from build123d import *

# Parameters (mm, degrees)
EXTRUDE_1_DEPTH              = 2.5
HOLE_WIZARD_M3_1_D           = 2.5
HOLE_WIZARD_M3_1_CSINK_D     = 3.05
HOLE_WIZARD_M3_1_CSINK_ANGLE = 90
SKETCH_8_W                   = 27.92487284
SKETCH_8_H                   = 6.74765502
SKETCH_8_W_2                 = 35.307317085
SKETCH_8_H_2                 = 2.5392143
SKETCH_8_W_3                 = 43.206671158
EXTRUDE_2_DEPTH              = 6
SKETCH_9_W                   = 15
SKETCH_9_H                   = 12
EXTRUDE_3_DEPTH              = 10.5
SKETCH_10_W                  = 2.54775384
SKETCH_10_H                  = 5.1401971
CUT_EXTRUDE_1_DEPTH          = 10.5
SKETCH_12_W                  = 14
SKETCH_12_H                  = 10
EXTRUDE_4_DEPTH              = 10
SKETCH_13_W                  = 10
SKETCH_13_H                  = 10
SKETCH_13_R                  = 2.75
EXTRUDE_5_DEPTH              = 3.5
SKETCH_14_R                  = 2.75
CUT_EXTRUDE_3_DEPTH          = 8


with BuildPart() as part:
    # 草图1 → 凸台-拉伸1 (new body)
    with BuildSketch(Plane.XY):
        Polygon((-35.4452235, 28.536703393), (-35.4452235, -24.463296607), (30.5947765, -24.463296607), (30.5947765, -20.997866899), (34.409346792, -17.183296607), (34.409346792, 10.756703393), (30.5947765, 14.571273684), (30.5947765, 28.536703393), align=None)
    extrude(amount=EXTRUDE_1_DEPTH)

    # M3 螺纹孔1 (through all)
    with Locations(Plane.XY.offset(2.5)):
        with Locations((-20.2052235, 25.996703393), (30.5947765, 10.756703393), (30.5947765, -17.183296607), (-20.2052235, -22.263296607)):
            CounterSinkHole(HOLE_WIZARD_M3_1_D / 2, HOLE_WIZARD_M3_1_CSINK_D / 2, counter_sink_angle=HOLE_WIZARD_M3_1_CSINK_ANGLE)

    # 草图8 → 凸台-拉伸2 (add)
    with BuildSketch(Plane.XY.offset(2.5)):
        with Locations((7.351969456, -11.104054762)):
            Rectangle(SKETCH_8_W, SKETCH_8_H)
        with Locations((7.55461376, -21.179250047)):
            Rectangle(SKETCH_8_W_2, SKETCH_8_H_2)
        with Locations((5.71151473, 24.713414732)):
            Rectangle(SKETCH_8_W_3, SKETCH_8_H_2)
    extrude(amount=EXTRUDE_2_DEPTH)

    # 草图9 → 凸台-拉伸3 (add)
    with BuildSketch(Plane.XY.offset(2.5)):
        with Locations((-33.9452235, 12.536703393)):
            Rectangle(SKETCH_9_W, SKETCH_9_H)
    extrude(amount=EXTRUDE_3_DEPTH)

    # 草图10 → 切除-拉伸1 (cut)
    with BuildSketch(Plane.ZY.offset(41.4452235)):
        Polygon((3.5, 17.344772898), (3.5, 7.728633887), (9.323306646, 7.728633887), (12, 9.706966862), (12, 15.452627596), (9.323306646, 17.344772898), align=None)
        with Locations((7.507872917, 12.536703393)):
            Rectangle(SKETCH_10_W, SKETCH_10_H, mode=Mode.SUBTRACT)
    extrude(amount=-CUT_EXTRUDE_1_DEPTH, mode=Mode.SUBTRACT)

    # 草图12 → 凸台-拉伸4 (add)
    with BuildSketch(Plane.XY.offset(2.5)):
        with Locations((-28.4452235, -13.463296607)):
            Rectangle(SKETCH_12_W, SKETCH_12_H)
    extrude(amount=EXTRUDE_4_DEPTH)

    # 草图13 → 凸台-拉伸5 (add)
    with BuildSketch(Plane.ZY.offset(35.4452235)):
        with Locations((7.5, -13.463296607)):
            Rectangle(SKETCH_13_W, SKETCH_13_H)
        with Locations((7.5, -13.463296607)):
            Circle(SKETCH_13_R, mode=Mode.SUBTRACT)
    extrude(amount=EXTRUDE_5_DEPTH)

    # 草图14 → 切除-拉伸3 (cut)
    with BuildSketch(Plane.ZY.offset(35.4452235)):
        with Locations((7.5, -13.463296607)):
            Circle(SKETCH_14_R)
    extrude(amount=-CUT_EXTRUDE_3_DEPTH, mode=Mode.SUBTRACT)


solid = part.part
Read the model definition and answer for the solid it produces. Units are mm, in the model's axes. A direction names the side the tool comes from. Round coordinates to 2 decimals unless told otherwise and drop trailing zeros. Write each loop counter-clockwise with the first axis right and the second up, starting at its lowest first coordinate (ties: lowest second). Pieces come first, ordered by that corner, then holes.
1. The part is cut by section C-C, the plane z = 11.25. Determine the outline of the cut face in (x, y), then the cut area to 3 significant figures.
2. The part is cut by section A-A, the plane z = 7.5. State how many separate pieces and enclosed holes the cut face has, then the cut area to 3 significant figures.
3. Which of the six approach directions +Z, -Z, +X, -X, +Y, -Y give full straight-line access (tool end or side, diameter ignored) to faces 5 (the face through (-38.945, -11, 10)), 6 (the face through (-33.11, -14.52, 10.04)), 7 (the face through (-10.099, -21, 5)), 8 (the face through (-34, 6.537, 8))?
4. Determine the mould class of faces 1 (the face through (-30, -8.463, 7)), 2 (the face through (-38, 13, 2.5)), 3 (the face through (-36, 7.729, 6)), 4 (the face through (-36, 13, 3.5)) for opening direction Z: pulls with the +Z half, pulls with the -Z half, needs draft (parallel to the pull), parting line crosses it, or undercut.
5. Straight lines are drawn through the part: L1, parallel to Y at x = -31.5, z = 4.5; L2, parallel to Y at x = -32, z = 7.5; L3, parallel to Y at x = 3, z = 4. For each, find the intervals that lie inside material, in ascending order.
6. The part is cut by section B-B, the plane x = -2.5. Determine the outline of the cut face in (y, z).
7. Given pin 1 Ø6.5 at (x, z) = (13.5, 4) entering from -Y; pin 2 Ø1.3 at (y, z) = (-20.5, 6) entering from +X; pin 3 Ø3 at (x, z) = (9, 5.5) entering from +Y; pin 4 Ø3 at (y, z) = (22.5, 1) entering from +X, each flat-ended and moving along its own axis, determine where each tip first touches the part or whether it passes through.
8. The part is cut by section D-D, the plane y = -5. Determine the outline of the cut face in (x, z), then the cut area to 3 significant figures.
Values:
1. outline: (-41.45, 6.54) - (-26.45, 6.54) - (-26.45, 18.54) - (-41.45, 18.54) - (-41.45, 15.98) - (-30.95, 15.98) - (-30.95, 9.15) - (-41.45, 9.15) - close; (-38.95, -18.46) - (-21.45, -18.46) - (-21.45, -8.46) - (-38.95, -8.46) - close
1. area: 283 mm2
2. separate pieces: 5
2. enclosed holes: 0
2. area: 633 mm2
3. face 5: +Z, -Z, -X, -Y
3. face 6: -X
3. face 7: +Z, -X, -Y
3. face 8: +Z, +X, -X
4. face 1: needs draft
4. face 2: pulls with the -Z half
4. face 3: undercut
4. face 4: undercut
5. L1: y = -18.46 to -8.46, 6.54 to 7.73, 17.34 to 18.54
5. L2: y = -18.46 to -16.21, -10.71 to -8.46, 6.54 to 7.73, 9.97 to 15.11, 17.34 to 18.54
5. L3: y = -22.45 to -19.91, -14.48 to -7.73, 23.44 to 25.98
6. outline: (-24.46, 0) - (28.54, 0) - (28.54, 2.5) - (25.98, 2.5) - (25.98, 8.5) - (23.44, 8.5) - (23.44, 2.5) - (-7.73, 2.5) - (-7.73, 8.5) - (-14.48, 8.5) - (-14.48, 2.5) - (-19.91, 2.5) - (-19.91, 8.5) - (-22.45, 8.5) - (-22.45, 2.5) - (-24.46, 2.5) - close
7. pin 1: stops at y = -24.46
7. pin 2: stops at x = 25.21
7. pin 3: stops at y = 25.98
7. pin 4: stops at x = 30.59
8. outline: (-35.45, 0) - (34.41, 0) - (34.41, 2.5) - (-35.45, 2.5) - close
8. area: 175 mm2
